```python
from build123d import *

# Parameters (mm, degrees)
SKETCH1_W           = 88.9
SKETCH1_H           = 88.9
SKETCH1_R           = 2.032
SKETCH1_W_2         = 63.5
SKETCH1_H_2         = 63.5
SKETCH1_W_3         = 50.8
SKETCH1_H_3         = 50.8
BOSS_EXTRUDE2_DEPTH = 3.175


with BuildPart() as part:
    # Sketch1 → Boss-Extrude2 (new body)
    with BuildSketch(Plane(origin=(0, 0, 0), x_dir=(1, 0, 0), z_dir=(0, 1, 0))):
        Rectangle(SKETCH1_W, SKETCH1_H)
        with Locations(Location((38.1, 38.1, 0), (0, 0, 270))):
            Circle(SKETCH1_R, mode=Mode.SUBTRACT)
        with Locations(Location((-38.1, 38.1, 0), (0, 0, 270))):
            Circle(SKETCH1_R, mode=Mode.SUBTRACT)
        with Locations(Location((38.1, -38.1, 0), (0, 0, 270))):
            Circle(SKETCH1_R, mode=Mode.SUBTRACT)
        with Locations(Location((-38.1, -38.1, 0), (0, 0, 270))):
            Circle(SKETCH1_R, mode=Mode.SUBTRACT)
        Rectangle(SKETCH1_W_2, SKETCH1_H_2, mode=Mode.SUBTRACT)
        Rectangle(SKETCH1_W_2, SKETCH1_H_2)
        Rectangle(SKETCH1_W_3, SKETCH1_H_3, mode=Mode.SUBTRACT)
        Rectangle(SKETCH1_W_3, SKETCH1_H_3)
    extrude(amount=BOSS_EXTRUDE2_DEPTH)


solid = part.part
```
The model under review builds one solid part; all positions refer to its coordinate system, in mm. Round coordinates to 2 decimals unless told otherwise and drop trailing zeros. Write each loop counter-clockwise with the first axis right and the second up, starting at its lowest first coordinate (ties: lowest second). Pieces come first, ordered by that corner, then holes. Notation, with made-up numbers: (53, 73) -> (79, 73) arc R10 cw to (79, 79) -> close; hole circle Ø9 at (-40, 24). An arc over 180 degrees is marked (long way). Use CSV: the item, a comma, the result in double quotes.
Q1. Consider section B-B (x = 38.1). Give the boundary of the cut face in (y, z) (3 decimals).
Checks:
outline,"(0, -44.45) -> (3.175, -44.45) -> (3.175, -40.132) -> (0, -40.132) -> close; (0, -36.068) -> (3.175, -36.068) -> (3.175, 36.068) -> (0, 36.068) -> close; (0, 40.132) -> (3.175, 40.132) -> (3.175, 44.45) -> (0, 44.45) -> close"
Q2. To check wall thickness, follow probe 1 along X at (y, z) = (2.5, 38.1); probe 2 along X at (y, z) = (0.4, 36.5). State the ranges of each line that lie inside material, in increasing order. Write a range as [from, to].
Checks:
probe 1,"[-44.45, -40.13], [-36.07, 36.07], [40.13, 44.45]"
probe 2,"[-44.45, -39.35], [-36.85, 36.85], [39.35, 44.45]"
Q3. For pin 1 Ø3.5 at (x, z) = (-38.1, 38.1) entering from -Y (3 decimals), flat-tipped, find the tip position at first contact; note if it passes through.
Checks:
pin 1,"through"
Q4. Consider section A-A (z = -38.1). Give the boundary of the cut face in (x, y) (3 decimals).
Checks:
outline,"(-44.45, 0) -> (-40.132, 0) -> (-40.132, 3.175) -> (-44.45, 3.175) -> close; (-36.068, 0) -> (36.068, 0) -> (36.068, 3.175) -> (-36.068, 3.175) -> close; (40.132, 0) -> (44.45, 0) -> (44.45, 3.175) -> (40.132, 3.175) -> close"
Q5. Mouldability with a two-part tool opening along Z and no side actions: class faces 1 (the flat face through (44.45, 2, 1)), 2 (the cylindrical face through (-39.34, 1.57, 36.49)), 3 (the flat face through (-1, 2, 44.45)), 4 (the cylindrical face through (39.47, 1.57, 36.6)) as released by +Z, released by -Z, zero draft, split by the parting line, or undercut.
Checks:
face 1,"zero draft"
face 2,"undercut"
face 3,"released by +Z"
face 4,"undercut"
